Study the drawing (mm; zero at the part's minimum x, y, z) and answer. A direction names the side the tool comes from. Coordinates: 2 decimals unless noted, no trailing zeros. Write each loop counter-clockwise with the first axis right and the second up, starting at its lowest first coordinate (ties: lowest second). Pieces come first, ordered by that corner, then holes. Notation, with made-up numbers: (74, 48.25) - (84, 48.25) arc R34 cw to (84, 83.25) - close; hole circle Ø1 at (55.5, 18.5). An arc over 180 degrees is marked (long way). One line per item, written item: value.
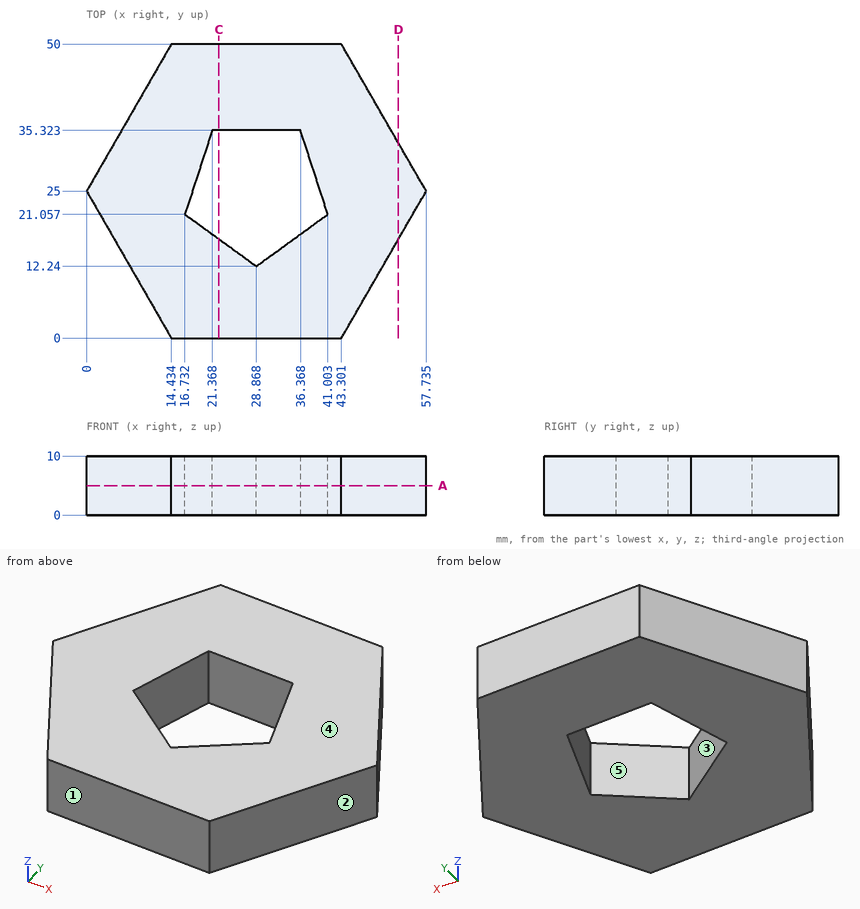
Item 1: Section C-C, the plane x = 22.5 is taken. Determine the outline of the cut face in (y, z).
Evaluation:
outline: (0, 0) - (16.87, 0) - (16.87, 10) - (0, 10) - close; (35.32, 0) - (50, 0) - (50, 10) - (35.32, 10) - close
Item 2: Determine the mould class of the marked faces 1, 2 and 3 for opening direction X: +X half, -X half, draft (parallel to the pull), parting line (faces both ways), or undercut.
Evaluation:
face 1: draft
face 2: +X half
face 3: undercut
Item 3: Given pin 1 (10 mm diameter, centred on x = 13, y = 15, fed in from -Z); pin 2 (1 mm diameter, centred on y = 8.5, z = 8.5, fed in from -X); pin 3 (4 mm diameter, centred on y = 17.5, z = 3.5, fed in from -X) (1 decimal); pin 4 (5 mm diameter, centred on x = 47, z = 2, fed in from +Y) (1 decimal), each flat-ended and moving along its own axis, determine where each tip first touches the part or whether it passes through.
Evaluation:
pin 1: stops at z = 0
pin 2: stops at x = 9.24
pin 3: stops at x = 3.2
pin 4: stops at y = 47.9
Item 4: Which of the six approach directions +Z, -Z, +X, -X, +Y, -Y give full straight-line access (tool end or side, diameter ignored) to the marked faces 4 and 5?
Evaluation:
face 4: +Z, +X, -X, +Y, -Y
face 5: +Z, -Z
Item 5: Consider probe 1 along X at (y, z) = (13.5, 2) (1 decimal); probe 2 along X at (y, z) = (31.5, 6.75) (1 decimal); probe 3 along Y at (x, z) = (34, 5.75) (1 decimal). Determine where each line is inside the solid, lowest interval first.
Evaluation:
probe 1: x = 6.6 to 27.1, 30.6 to 51.1
probe 2: x = 3.8 to 20.1, 37.6 to 54
probe 3: y = 0 to 16, 35.3 to 50
Item 6: Section A-A, the plane z = 5 is taken. Determine the outline of the cut face in (x, y) (1 decimal), then the cut area to 3 significant figures.
Evaluation:
outline: (0, 25) - (14.4, 0) - (43.3, 0) - (57.7, 25) - (43.3, 50) - (14.4, 50) - close; hole (16.7, 21.1) - (28.9, 12.2) - (41, 21.1) - (36.4, 35.3) - (21.4, 35.3) - close
area: 1,780 mm2
Item 7: Section D-D, the plane x = 53 is taken. Determine the outline of the cut face in (y, z).
Evaluation:
outline: (16.8, 0) - (33.2, 0) - (33.2, 10) - (16.8, 10) - close
